from build123d import *

# Parameters (mm, degrees)
BOSS_EXTRUDE1_DEPTH = 40
FILLET1_R           = 5
FILLET2_R           = 5


with BuildPart() as part:
    # Sketch1 → Boss-Extrude1 (new body)
    with BuildSketch(Plane.XY):
        Polygon((0, 0), (34.925, 0), (34.925, -34.925), (38.1, -34.925), (38.1, 0), (38.1, 3.175), (0, 3.175), align=None)
    extrude(amount=BOSS_EXTRUDE1_DEPTH)

    # Fillet1
    fillet1_edges = [part.edges().sort_by_distance(p)[0] for p in [
        (34.925, 0, 20),
    ]]
    fillet(fillet1_edges, radius=FILLET1_R)

    # Fillet2
    fillet2_edges = [part.edges().sort_by_distance(p)[0] for p in [
        (38.1, 3.175, 20),
    ]]
    fillet(fillet2_edges, radius=FILLET2_R)


solid = part.part
Work out the finished part from the listing and answer in its coordinate system (mm). A direction names the side the tool comes from. Give positions to 0.01 mm unless a question says otherwise; leave off trailing zeros. Write each loop counter-clockwise with the first axis right and the second up, starting at its lowest first coordinate (ties: lowest second). Pieces come first, ordered by that corner, then holes. Notation, with made-up numbers: M 59,-12.5 L 98,-12.5 A21 ccw 98,-2.5 Z; hole C -3,-21 d2. An arc over 180 degrees is marked long. Answer as CSV lines item,"result".
Q1. A tool of negligible diameter and unlimited length cuts with its end or side. For faces 1 (the flat face through (36, -34.925, 20)), 2 (the flat face through (34.925, -20, 20)), from which of +Z, -Z, +X, -X, +Y, -Y can it reach the whole face along a straight path? Write none if from no direction.
A:
face 1,"+Z, -Z, +X, -X, -Y"
face 2,"+Z, -Z, -X, -Y"
Q2. A cutting plane is placed at A-A on z = 18.5. Write down the section's boundary in (x, y) (3 decimals).
A:
outline,"M 0,0 L 29.925,0 A5 cw 34.925,-5 L 34.925,-34.925 L 38.1,-34.925 L 38.1,-1.825 A5 ccw 33.1,3.175 L 0,3.175 Z"
Q3. Given P1, Ø15, axis at x = 16.5, z = 25, coming from the -Y side; P2, Ø4, axis at y = -14.5, z = 26, coming from the -X side (3 decimals), each flat-ended and moving along its own axis, determine where each tip first touches the part or whether it passes through.
A:
P1,"stops at y = 0"
P2,"stops at x = 34.925"
Q4. A cutting plane is placed at C-C on x = 14.5. Write down the section's boundary in (y, z) (3 decimals).
A:
outline,"M 0,0 L 3.175,0 L 3.175,40 L 0,40 Z"
Q5. A cutting plane is placed at B-B on y = -28.5. Write down the section's boundary in (x, z) (3 decimals).
A:
outline,"M 34.925,0 L 38.1,0 L 38.1,40 L 34.925,40 Z"
Q6. Find the intervals of material crossed by probe 1 along Y at (x, z) = (3.5, 38) (3 decimals); probe 2 along X at (y, z) = (-26, 7.5) (3 decimals); probe 3 along Y at (x, z) = (32.5, 2) (3 decimals), in increasing order. Write a range as [from, to].
A:
probe 1,"y = [0, 3.175]"
probe 2,"x = [34.925, 38.1]"
probe 3,"y = [-0.714, 3.175]"
